from build123d import *

# Parameters (mm, degrees)
SKETCH_R         = 11.5
PAD_DEPTH        = 6.4002
HOLE_D           = 5.0292
HOLE_CBORE_D     = 8.4248
HOLE_CBORE_DEPTH = 2.4002
SKETCH002_W      = 4
SKETCH002_H      = 7.112352
PAD001_DEPTH     = 25
CHAMFER_ANGLE    = 45
CHAMFER_SIZE     = 5
SKETCH003_R      = 0.95
POCKET_DEPTH     = 4.5
POCKET001_DEPTH  = 6.4012


with BuildPart() as part:
    # Sketch → Pad (new body)
    with BuildSketch(Plane.XY):
        Circle(SKETCH_R)
    extrude(amount=PAD_DEPTH)

    # Hole (through all)
    with Locations(Plane.XY.offset(6.4002)):
        with Locations((0, 0)):
            CounterBoreHole(HOLE_D / 2, HOLE_CBORE_D / 2, HOLE_CBORE_DEPTH)

    # Sketch002 (on DatumPlane) → Pad001 (join)
    with BuildSketch(Plane.XY.offset(6.4002)):
        with Locations((0, -7.768576)):
            Rectangle(SKETCH002_W, SKETCH002_H)
    extrude(amount=PAD001_DEPTH)

    # Chamfer
    chamfer_edges = [part.edges().sort_by_distance(p)[0] for p in [
        (0, -11.324752, 31.4002),
    ]]
    chamfer_side = part.faces().sort_by_distance((0, -11.324752, 18.9002))[0]
    chamfer(chamfer_edges, length=CHAMFER_SIZE, angle=CHAMFER_ANGLE, reference=chamfer_side)

    # Sketch003 (on Face3 of Chamfer) → Pocket (cut)
    with BuildSketch(Plane(origin=(0, -18.862476, 18.862476), x_dir=(1, 0, 0), z_dir=(0, -0.707107, 0.707107))):
        with Locations((0, 13.209952)):
            Circle(SKETCH003_R)
    extrude(amount=-POCKET_DEPTH, mode=Mode.SUBTRACT)

    # Sketch004 (on DatumPlane) → Pocket001 (cut, through all)
    with BuildSketch(Plane.XY.offset(6.4002)):
        with BuildLine():
            ThreePointArc((-2, -11.324752), (0, -11.5), (2, -11.324752))
            Line((-2, -11.324752), (2, -11.324752))
        make_face()
    extrude(amount=-POCKET001_DEPTH, mode=Mode.SUBTRACT)


solid = part.part
Geometry: final body of the model. Coordinates: model frame, mm. A direction names the side the tool comes from. Coordinates: 2 decimals unless noted, no trailing zeros. Loops run counter-clockwise (first coordinate to the right, second up) from the corner with the lowest first, then second, coordinate; pieces in that order, holes last. Notation, with made-up numbers: M 20.5,1 L 77.5,1 A20 cw 77.5,35 Z; hole C 77,-3.5 d4. An arc over 180 degrees is marked long. One line per item, written item: value. Start each with the question number.
1) Reachability of faces 5 (the flat face through (0, -4.212, 19)), 6 (the flat face through (2, -8, 19)), 7 (the flat face through (2, -2, 4)), 8 (the flat face through (0, -11.325, 13)) from +Z, -Z, +X, -X, +Y, -Y: full face, straight path, thin tool, end or side. Return the list, or none.
2) Cut plane A-A (y = 0). Return loops of the section in (x, z).
3) Pin query (flat end, axial travel): P1, Ø3, axis at x = 5, z = 25.5, coming from the +Y side; P2, Ø3, axis at y = -5, z = 9.5, coming from the +X side; P3, Ø2, axis at x = 4, z = 5.5, coming from the -Y side; P4, Ø4, axis at x = 1.5, y = 0.5, coming from the +Z side. Return the tip coordinate at first contact, or that it passes through.
4) Material intervals for L1, parallel to Y at x = 0, z = 5.45; L2, parallel to X at y = 0, z = 4.5; L3, parallel to Y at x = 0, z = 2.8, sorted ascending. Write a range as from..to.
5) Draft query along Z for faces 1 (the flat face through (-2, -8, 19)), 2 (the cylindrical face through (0.511, -7.386, 27.201)), 3 (the flat face through (-0.01, -6.33, 25.03)), 4 (the flat face through (0, -5, 31.4)). Return one class per face: released by +Z, released by -Z, zero draft, split by the parting line, or undercut.
6) Cut plane C-C (z = 10). Return loops of the section in (x, y).
7) Cut plane D-D (y = -3.25). Return loops of the section in (x, z), then the cut area to 3 significant figures.
Evaluation:
1. face 5: +Z, +X, -X, +Y
1. face 6: +Z, +X, +Y, -Y
1. face 7: +Z
1. face 8: +Z, -Z, +X, -X, -Y
2. outline: M -11.5,0 L -2.51,0 L -2.51,4 L -4.21,4 L -4.21,6.4 L -11.5,6.4 Z; M 2.51,0 L 11.5,0 L 11.5,6.4 L 4.21,6.4 L 4.21,4 L 2.51,4 Z
3. P1: through
3. P2: x = 2
3. P3: y = -11.1
3. P4: z = 4
4. L1: -11.32..-4.21, 4.21..11.5
4. L2: -11.5..-4.21, 4.21..11.5
4. L3: -11.32..-2.51, 2.51..11.5
5. face 1: zero draft
5. face 2: undercut
5. face 3: undercut
5. face 4: released by +Z
6. outline: M -2,-11.32 L 2,-11.32 L 2,-4.21 L -2,-4.21 Z
7. outline: M -11.03,0 L 11.03,0 L 11.03,6.4 L 2.68,6.4 L 2.68,4 L -2.68,4 L -2.68,6.4 L -11.03,6.4 Z
7. area: 128 mm^2
